```python
from build123d import *

# Parameters (mm, degrees)
BOSS_EXTRUDE1_DEPTH = 1.5
SKETCH2_R           = 1.25
CUT_EXTRUDE1_DEPTH  = 27.911893282
SKETCH3_W           = 4
SKETCH3_H           = 6
BOSS_EXTRUDE2_DEPTH = 3
SKETCH4_W           = 0.314102564
SKETCH4_H           = 3.5
CUT_EXTRUDE2_DEPTH  = 0.5


with BuildPart() as part:
    # Sketch1 → Boss-Extrude1 (new body)
    with BuildSketch(Plane.XY):
        with BuildLine():
            Line((3, 0), (16, 0))
            ThreePointArc((16, 0), (16.707106781, 0.292893219), (17, 1))
            Line((17, 1), (17, 4))
            ThreePointArc((17, 4), (17.367006838, 5.154700538), (18.333333333, 5.885618083))
            ThreePointArc((18.333333333, 5.885618083), (18.816496581, 6.251076856), (19, 6.828427125))
            Line((19, 6.828427125), (19, 18))
            ThreePointArc((19, 18), (18.707106781, 18.707106781), (18, 19))
            Line((18, 19), (1, 19))
            ThreePointArc((1, 19), (0.292893219, 18.707106781), (0, 18))
            Line((0, 18), (0, 6.828427125))
            ThreePointArc((0, 6.828427125), (0.183503419, 6.251076856), (0.666666667, 5.885618083))
            ThreePointArc((0.666666667, 5.885618083), (1.632993162, 5.154700538), (2, 4))
            Line((2, 4), (2, 1))
            ThreePointArc((2, 1), (2.292893219, 0.292893219), (3, 0))
        make_face()
    extrude(amount=BOSS_EXTRUDE1_DEPTH)

    # Sketch2 → Cut-Extrude1 (cut, through all)
    with BuildSketch(Plane(origin=(0, 0, 0), x_dir=(-1, 0, 0), z_dir=(0, 0, -1))):
        with Locations((-16.75, 16.75)):
            Circle(SKETCH2_R)
    cut_extrude1 = extrude(amount=-CUT_EXTRUDE1_DEPTH, mode=Mode.SUBTRACT)

    # Mirror1: Cut-Extrude1 across plane
    add(cut_extrude1.mirror(Plane.ZY.offset(-9.5)), mode=Mode.SUBTRACT)

    # Sketch3 → Boss-Extrude2 (add)
    with BuildSketch(Plane(origin=(0, 0, 0), x_dir=(-1, 0, 0), z_dir=(0, 0, -1))):
        with Locations((-15.652122357, 10)):
            Rectangle(SKETCH3_W, SKETCH3_H)
    extrude(amount=BOSS_EXTRUDE2_DEPTH)

    # Sketch4 → Cut-Extrude2 (cut)
    with BuildSketch(Plane(origin=(0, 0, 0), x_dir=(-1, 0, 0), z_dir=(0, 0, -1))):
        with Locations((-14.095226395, 2.323572114)):
            Rectangle(SKETCH4_W, SKETCH4_H)
        Polygon((-13.220226395, 0.573572114), (-12.758187132, 4.073572114), (-12.713315337, 4.073572114), (-11.268303318, 1.201777242), (-9.82749803, 4.073572114), (-9.782626235, 4.073572114), (-9.316380241, 0.573572114), (-9.630482805, 0.573572114), (-9.967021267, 3.089898236), (-11.229741619, 0.573572114), (-11.301256042, 0.573572114), (-12.569585369, 3.097610576), (-12.904020466, 0.573572114), align=None)
        with BuildLine():
            Line((-8.598431523, 4.073572114), (-8.284328959, 4.073572114))
            Line((-8.284328959, 4.073572114), (-8.284328959, 1.976516826))
            add(Edge.make_bspline(
                [(-8.284328959, 1.976516826), (-8.284375703, 1.94683609), (-8.284464408, 1.890511779), (-8.283871894, 1.810343478), (-8.282212526, 1.739071019), (-8.281166366, 1.676419672), (-8.278839032, 1.622676924), (-8.276940986, 1.577551614), (-8.274500429, 1.541257411), (-8.271567311, 1.520076485), (-8.270306523, 1.510971954)],
                knots=[0, 0, 0, 0, 1.528628734, 2.90083645, 4.128790002, 5.200304208, 6.127813768, 6.898992206, 7.526736466, 8, 8, 8, 8], degree=3))
            add(Edge.make_bspline(
                [(-8.270306523, 1.510971954), (-8.265129064, 1.478125191), (-8.255065878, 1.414282461), (-8.2294195, 1.32337418), (-8.193601999, 1.241442721), (-8.151158957, 1.16593143), (-8.095226345, 1.09894207), (-8.02822281, 1.037230417), (-7.947045041, 0.983258613), (-7.856784436, 0.933907801), (-7.759499198, 0.894242719), (-7.660087932, 0.864249354), (-7.560044953, 0.845970454), (-7.493068788, 0.843853915), (-7.459809728, 0.842802883)],
                knots=[0, 0, 0, 0, 1.035780045, 2.013197591, 2.933192213, 3.817615948, 4.702609284, 5.640816605, 6.646850145, 7.73207398, 8.84249596, 9.914020372, 10.964143139, 12, 12, 12, 12], degree=3))
            add(Edge.make_bspline(
                [(-7.459809728, 0.842802883), (-7.431255988, 0.843876734), (-7.374313426, 0.846018232), (-7.289706995, 0.859279663), (-7.207306887, 0.883180229), (-7.126706207, 0.914019987), (-7.051155222, 0.954767578), (-6.98061178, 1.001838418), (-6.917647846, 1.057049294), (-6.860189848, 1.118149638), (-6.810154912, 1.187089438), (-6.766783771, 1.262367576), (-6.731257841, 1.345116923), (-6.713714316, 1.403271345), (-6.704701555, 1.433147435)],
                knots=[0, 0, 0, 0, 0.994687771, 1.983630487, 2.973142513, 3.978332533, 4.983357753, 5.956394766, 6.925816176, 7.893390482, 8.871859704, 9.88551698, 10.913711441, 12, 12, 12, 12], degree=3))
            add(Edge.make_bspline(
                [(-6.704701555, 1.433147435), (-6.70170143, 1.445496009), (-6.695015942, 1.473013609), (-6.688768897, 1.5195349), (-6.682262371, 1.574424264), (-6.677747801, 1.638076076), (-6.673346581, 1.710277049), (-6.670713508, 1.791403307), (-6.669496475, 1.881160267), (-6.669133795, 1.943797429), (-6.668944344, 1.976516826)],
                knots=[0, 0, 0, 0, 0.558680831, 1.244966039, 2.062412453, 2.990489873, 4.051219941, 5.244515665, 6.560634259, 8, 8, 8, 8], degree=3))
            Line((-6.668944344, 1.976516826), (-6.668944344, 4.073572114))
            Line((-6.668944344, 4.073572114), (-6.35484178, 4.073572114))
            Line((-6.35484178, 4.073572114), (-6.35484178, 1.959689903))
            add(Edge.make_bspline(
                [(-6.35484178, 1.959689903), (-6.3550959, 1.921591524), (-6.355591831, 1.847240221), (-6.359892408, 1.738288862), (-6.366749408, 1.63493588), (-6.376437496, 1.537167384), (-6.389274499, 1.445333225), (-6.403549719, 1.358628457), (-6.421729252, 1.277675464), (-6.442962654, 1.201843046), (-6.467236202, 1.129657533), (-6.49867735, 1.061148918), (-6.53410185, 0.994234519), (-6.576116503, 0.92992641), (-6.623327885, 0.867939856), (-6.676779566, 0.808650781), (-6.734703727, 0.751111735), (-6.798063287, 0.696798669), (-6.865813812, 0.646989992), (-6.93775377, 0.603192221), (-7.013330539, 0.566168604), (-7.092347666, 0.535692679), (-7.174838868, 0.51277808), (-7.260806228, 0.495702924), (-7.350445421, 0.486000627), (-7.411410078, 0.484558697), (-7.442281683, 0.483828524)],
                knots=[0, 0, 0, 0, 1.316592851, 2.569410997, 3.76748051, 4.895814652, 5.963796859, 6.97159953, 7.931736103, 8.829262218, 9.692595152, 10.560224239, 11.431080259, 12.30701507, 13.211635791, 14.121146779, 15.063487852, 16.031507147, 17.00238618, 17.966455255, 18.938106653, 19.907068911, 20.888905087, 21.893141452, 22.933117798, 24, 24, 24, 24], degree=3))
            add(Edge.make_bspline(
                [(-7.442281683, 0.483828524), (-7.475950786, 0.48461329), (-7.542009445, 0.486152996), (-7.639347512, 0.494975746), (-7.732661709, 0.511594141), (-7.822937586, 0.532754085), (-7.908946083, 0.561937822), (-7.991839527, 0.596035947), (-8.070198208, 0.637913207), (-8.145293337, 0.6845066), (-8.215118093, 0.736931238), (-8.279215496, 0.794071412), (-8.337691367, 0.855011789), (-8.389560063, 0.920412155), (-8.435680948, 0.989763862), (-8.475411161, 1.063263102), (-8.509524405, 1.140881418), (-8.527130972, 1.194834619), (-8.536031683, 1.222109774)],
                knots=[0, 0, 0, 0, 1.13879206, 2.234305948, 3.301075583, 4.341971843, 5.366689343, 6.369221514, 7.369726634, 8.367512178, 9.355451585, 10.318319045, 11.268648973, 12.207971039, 13.137398894, 14.081662264, 15.030215811, 16, 16, 16, 16], degree=3))
            add(Edge.make_bspline(
                [(-8.536031683, 1.222109774), (-8.541208842, 1.240742349), (-8.552438213, 1.281156818), (-8.564463511, 1.348043306), (-8.574572592, 1.425058224), (-8.584078151, 1.512206842), (-8.589687108, 1.609556709), (-8.594604547, 1.717065625), (-8.598466166, 1.834863587), (-8.598443394, 1.916918102), (-8.598431523, 1.959689903)],
                knots=[0, 0, 0, 0, 0.625038921, 1.35572334, 2.194682327, 3.136881307, 4.189498639, 5.346923369, 6.617055217, 8, 8, 8, 8], degree=3))
            Line((-8.598431523, 1.959689903), (-8.598431523, 4.073572114))
        make_face()
    extrude(amount=-CUT_EXTRUDE2_DEPTH, mode=Mode.SUBTRACT)


solid = part.part
```
For this review, take the finished solid that the model builds, in its own axes (mm). A direction names the side the tool comes from. Round coordinates to 2 decimals unless told otherwise and drop trailing zeros. Write each loop counter-clockwise with the first axis right and the second up, starting at its lowest first coordinate (ties: lowest second). Pieces come first, ordered by that corner, then holes. Notation, with made-up numbers: (39.5, 17) - (65.5, 17) arc R9 ccw to (65.5, 27) - close; hole circle Ø2 at (0.25, 62.25). An arc over 180 degrees is marked (long way). Put each result on its own line as item: value.
Q1. We need section D-D (x = 14.75). Give the boundary of the cut face in (y, z).
Solved:
outline: (0, 0) - (7, 0) - (7, -3) - (13, -3) - (13, 0) - (19, 0) - (19, 1.5) - (0, 1.5) - close
Q2. We need section C-C (y = 10.25). Give the boundary of the cut face in (x, z).
Solved:
outline: (0, 0) - (13.65, 0) - (13.65, -3) - (17.65, -3) - (17.65, 0) - (19, 0) - (19, 1.5) - (0, 1.5) - close
Q3. We need section B-B (x = 16.75). Give the boundary of the cut face in (y, z).
Solved:
outline: (0.34, 0) - (7, 0) - (7, -3) - (13, -3) - (13, 0) - (15.5, 0) - (15.5, 1.5) - (0.34, 1.5) - close; (18, 0) - (19, 0) - (19, 1.5) - (18, 1.5) - close
Q4. Insertion check: pin 1 Ø2 at (x, y) = (2, 11) entering from -Z; pin 2 Ø0.9 at (x, z) = (15.5, -1) entering from +Y; pin 3 Ø0.9 at (x, z) = (16.5, -1) entering from -Y. Each pin has a flat end and moves straight along its axis. Give the tip position at first contact, or say it passes through.
Solved:
pin 1: stops at z = 0
pin 2: stops at y = 13
pin 3: stops at y = 7
Q5. Wall thickness on probe 1 along Y at (x, z) = (15.5, -2.55); probe 2 along Z at (x, y) = (8.25, 15.5); probe 3 along Y at (x, z) = (16.75, 0.85): over which ranges is each line inside the solid? List them lowest first.
Solved:
probe 1: y = 7 to 13
probe 2: z = 0 to 1.5
probe 3: y = 0.34 to 15.5, 18 to 19
Q6. Mouldability with a two-part tool opening along X and no side actions: class faces 4 (the face through (1.6, 5.2, 0.7)), 5 (the face through (12, 2.66, 0.25)), 6 (the face through (17.652, 10, -1)) as released by +X, released by -X, zero draft, split by the parting line, or undercut.
Solved:
face 4: released by -X
face 5: undercut
face 6: released by +X
Q7. Machinability: for faces 1 (the face through (10.8, 1.8, 0.5)), 2 (the face through (13.652, 10, -1)), 3 (the face through (2, 3, 1)), which of the approach directions +Z, -Z, +X, -X, +Y, -Y give a long, thin tool a straight path to every point of the face, cutting with its end or side? Answer none if there is none.
Solved:
face 1: -Z
face 2: -Z, -X, +Y, -Y
face 3: +Z, -Z, -X, -Y
Q8. We need section A-A (y = 16.75). Give the boundary of the cut face in (x, z), and give its area (3 significant figures).
Solved:
outline: (0, 0) - (1, 0) - (1, 1.5) - (0, 1.5) - close; (3.5, 0) - (15.5, 0) - (15.5, 1.5) - (3.5, 1.5) - close; (18, 0) - (19, 0) - (19, 1.5) - (18, 1.5) - close
area: 21.0 mm2
